Can you work these out from the model? Positions are in its coordinate system, mm. Face numbers are marked on the shaded views. A direction names the side the tool comes from. Give positions to 0.01 mm unless a question says otherwise; leave off trailing zeros. Order: outer loops, then holes, each group sorted by start corner. A loop starts at its lowest first (then second) coordinate and runs counter-clockwise, first axis right, second up. Notation, with made-up numbers: M 30,2.5 L 48,2.5 A15 ccw 48,12.5 Z; hole C -10.75,65.25 d6. An arc over 180 degrees is marked long. Use a Markdown table: item, result. Add a question column.
from build123d import *

# Parameters (mm, degrees)
F1_DEPTH = 9
F2_W     = 3
F2_H     = 20
F3_DEPTH = 30
F4_R     = 2.5
F5_DEPTH = 10
F7_DEPTH = 10
F8_R     = 10.5
F9_DEPTH = 5


with BuildPart() as f1:
    # F0 (on Front) → F1 (new body)
    with BuildSketch(Plane.XZ):
        with BuildLine():
            ThreePointArc((16.09375, -11.873971995), (18.998355192, -6.25), (20, 0))
            ThreePointArc((20, 0), (18.998355192, 6.25), (16.09375, 11.873971995))
            ThreePointArc((16.09375, 11.873971995), (7.5, 0), (16.09375, -11.873971995))
        make_face()
        with BuildLine():
            ThreePointArc((16.09375, 11.873971995), (18.998355192, 6.25), (20, 0))
            ThreePointArc((20, 0), (18.998355192, -6.25), (16.09375, -11.873971995))
            ThreePointArc((16.09375, -11.873971995), (27.3287746247, -10.1261573413), (32.5, 0))
            ThreePointArc((32.5, 0), (27.3287746247, 10.1261573413), (16.09375, 11.873971995))
        make_face()
        with BuildLine():
            ThreePointArc((16.09375, -11.873971995), (7.5, 0), (16.09375, 11.873971995))
            ThreePointArc((16.09375, 11.873971995), (0, 20), (-16.09375, 11.873971995))
            ThreePointArc((-16.09375, 11.873971995), (-9.8738426587, 7.3287746247), (-7.5, 0))
            ThreePointArc((-7.5, 0), (-9.8738426587, -7.3287746247), (-16.09375, -11.873971995))
            ThreePointArc((-16.09375, -11.873971995), (0, -20), (16.09375, -11.873971995))
        make_face()
        with BuildLine():
            ThreePointArc((-7.5, 0), (-9.8738426587, 7.3287746247), (-16.09375, 11.873971995))
            ThreePointArc((-16.09375, 11.873971995), (-20, 0), (-16.09375, -11.873971995))
            ThreePointArc((-16.09375, -11.873971995), (-9.8738426587, -7.3287746247), (-7.5, 0))
        make_face()
        with BuildLine():
            ThreePointArc((-16.09375, -11.873971995), (-20, 0), (-16.09375, 11.873971995))
            ThreePointArc((-16.09375, 11.873971995), (-32.5, 0), (-16.09375, -11.873971995))
        make_face()
    extrude(amount=F1_DEPTH)

    # F2 (on face) → F3 (join)
    with BuildSketch(Plane(origin=(0, 0, 0), x_dir=(-1, 0, 0), z_dir=(0, 1, 0))):
        with Locations((-3, 0)):
            Rectangle(F2_W, F2_H)
        with Locations((3, 0)):
            Rectangle(F2_W, F2_H)
    extrude(amount=F3_DEPTH)

    # F4 (on face) → F5 (cut)
    with BuildSketch(Plane(origin=(-4.5, 0, 0), x_dir=(0, -1, 0), z_dir=(-1, 0, 0))):
        with Locations((-22.5, 0)):
            Circle(F4_R)
    extrude(amount=-F5_DEPTH, mode=Mode.SUBTRACT)

    # F6 (on face) → F7 (cut)
    with BuildSketch(Plane(origin=(-4.5, 0, 0), x_dir=(0, -1, 0), z_dir=(-1, 0, 0))):
        with BuildLine():
            ThreePointArc((-22.3790090531, -10), (-29.9486686635, 0.115669367), (-22.0793280751, 10))
            Line((-22.0793280751, 10), (-30, 10))
            Line((-30, 10), (-30, -10))
            Line((-30, -10), (-22.3790090531, -10))
        make_face()
    extrude(amount=-F7_DEPTH, mode=Mode.SUBTRACT)

    # F8 (on face) → F9 (cut)
    with BuildSketch(Plane.XZ.offset(9)):
        with Locations((-20, 0)):
            Circle(F8_R)
        with Locations((20, 0)):
            Circle(F8_R)
    extrude(amount=-F9_DEPTH, mode=Mode.SUBTRACT)


solid = f1.part
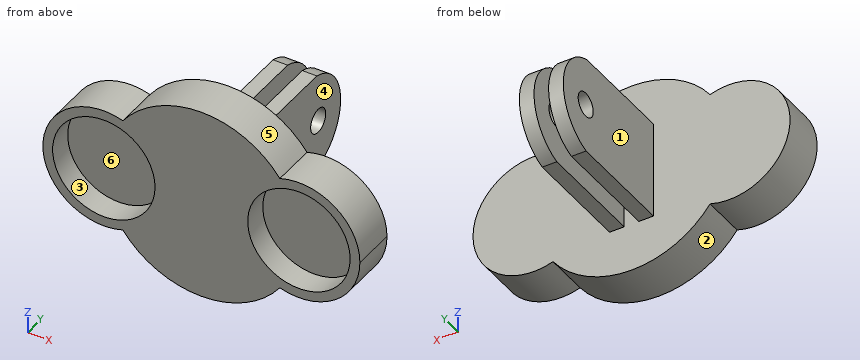
1. We'd pull the mould along Z, two halves only. Please class the marked faces 1, 2 and 3: +Z half, -Z half, draft (parallel to the pull), parting line (faces both ways), or undercut.
2. On a 3-axis mill with a long thin cutter (end or side, diameter ignored), from which of +Z, -Z, +X, -X, +Y, -Y can I reach the whole of each face in a straight line? I mean the marked faces 4, 5 and 6. Say none if no direction works.
3. If we section it at A-A, the plane y = 5: List the corners of the cut face in (x, z) for me.
4. If we section it at B-B, the plane x = 3: List the corners of the cut face in (y, z) for me, then the cut area to 3 significant figures.
5. Will these pins go through, and if not, where does the flat tip stop? pin 1 (12 mm diameter, centred on y = 15.5, z = -3.5, fed in from +X); pin 2 (3 mm diameter, centred on y = 16, z = -10, fed in from -X); pin 3 (6 mm diameter, centred on x = -0.5, y = -1.5, fed in from +Z); pin 4 (10.5 mm diameter, centred on x = 15, z = -3, fed in from -Y).
6. I need wall thicknesses on L1, parallel to X at y = -7, z = 3.5; L2, parallel to X at y = 2.5, z = -2.5; L3, parallel to Z at x = 20, y = -7.25. Which ranges of each line are inside material? Lowest first, please. Write a range as [from, to].
7. If we section it at D-D, the plane y = -1: List the corners of the cut face in (x, z) for me.
8. If we section it at C-C, the plane x = -20: List the corners of the cut face in (y, z) for me, then the cut area to 3 significant figures.
Geometry results:
| question | item | result |
|---|---|---|
| 1 | face 1 | draft |
| 1 | face 2 | -Z half |
| 1 | face 3 | undercut |
| 2 | face 4 | +Z, -Z, +X, +Y |
| 2 | face 5 | +Z, +Y, -Y |
| 2 | face 6 | -Y |
| 3 | outline | M -4.5,-10 L -1.5,-10 L -1.5,10 L -4.5,10 Z; M 1.5,-10 L 4.5,-10 L 4.5,10 L 1.5,10 Z |
| 4 | outline | M -9,-19.77 L 0,-19.77 L 0,-10 L 22.38,-10 A10.34 ccw 22.08,10 L 0,10 L 0,19.77 L -9,19.77 Z; hole C 22.5,0 d5 |
| 4 | area | 895 mm^2 |
| 5 | pin 1 | stops at x = 4.5 |
| 5 | pin 2 | stops at x = -4.5 |
| 5 | pin 3 | stops at z = 20 |
| 5 | pin 4 | stops at y = -9 |
| 6 | L1 | x = [-32, -29.9], [-10.1, 10.1], [29.9, 32] |
| 6 | L2 | x = [-4.5, -1.5], [1.5, 4.5] |
| 6 | L3 | z = [-12.5, -10.5], [10.5, 12.5] |
| 7 | outline | M -16.09,-11.87 A20 ccw 16.09,-11.87 A12.5 ccw long 16.09,11.87 A20 ccw -16.09,11.87 A12.5 ccw long Z |
| 8 | outline | M -9,-12.5 L 0,-12.5 L 0,12.5 L -9,12.5 L -9,10.5 L -4,10.5 L -4,-10.5 L -9,-10.5 Z |
| 8 | area | 120 mm^2 |
